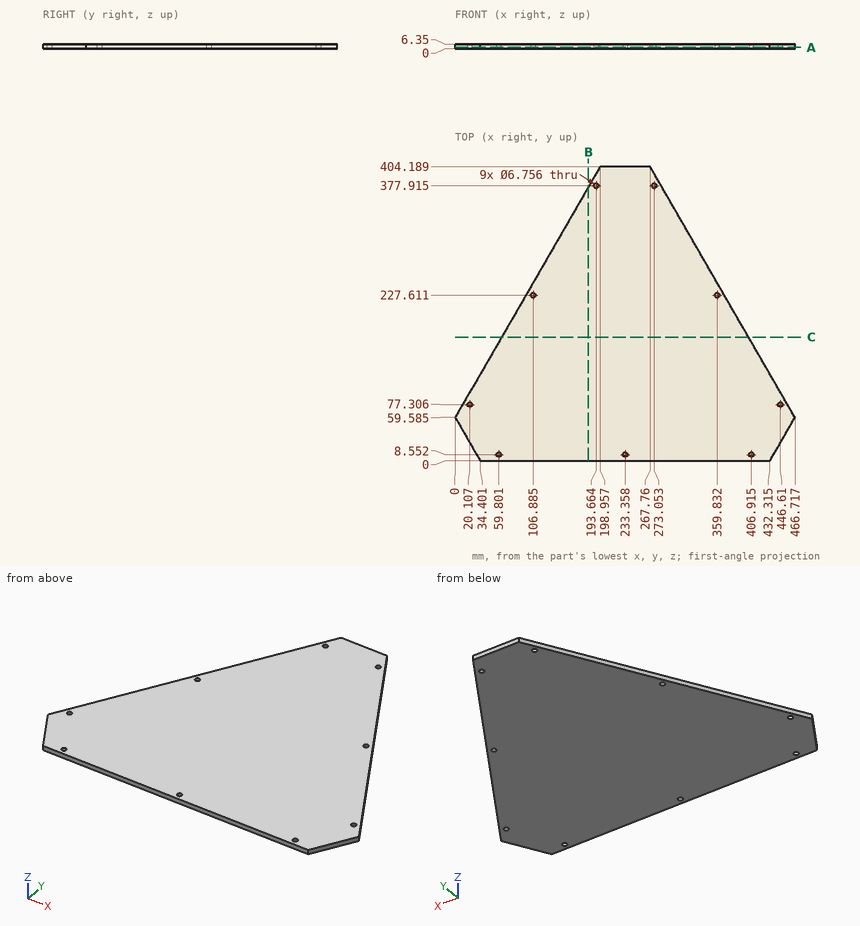
Drawing for the job (mm, zero at the part's lowest x, y, z). Give positions to 0.01 mm unless a question says otherwise; leave off trailing zeros. Loops run counter-clockwise (first coordinate to the right, second up) from the corner with the lowest first, then second, coordinate; pieces in that order, holes last. Notation, with made-up numbers: M 75.25,67 L 131.25,67 A26 cw 131.25,106 Z; hole C -34,67 d8. An arc over 180 degrees is marked long. Use one line per item in the form item = value.
Item 1: Slice it at B-B (x = 183). List the corners of the cut face in (y, z), plus the area to 3 significant figures.
Determined:
outline = M 0,0 L 376.55,0 L 376.55,6.35 L 0,6.35 Z
area = 2,390 mm2
Item 2: Drill centre lines: probe 1 along Y at (x, z) = (193, 5.75) (1 decimal); probe 2 along X at (y, z) = (142, 0.75) (1 decimal); probe 3 along X at (y, z) = (38, 1.25) (1 decimal). Where is each one in solid material? Low to high. Write a range as from..to.
Determined:
probe_1 = 0..374.6, 381.2..393.9
probe_2 = 47.6..419.1
probe_3 = 12.5..454.3
Item 3: Slice it at C-C (y = 170). List the corners of the cut face in (x, z), plus the area to 3 significant figures.
Determined:
outline = M 63.75,0 L 402.97,0 L 402.97,6.35 L 63.75,6.35 Z
area = 2,150 mm2
Item 4: Slice it at A-A (z = 1.75). Count the separate pieces of the cut face and the enclosed holes in it, plus the area to 3 significant figures.
Determined:
separate_pieces = 1
enclosed_holes = 9
area = 118,000 mm2
Item 5: Flat gauge pin, fed straight in: pin 1 (3 mm diameter, centred on x = 316, z = 1, fed in from +Y) (1 decimal). Where does the tip first touch, or does it go through?
Determined:
pin_1 = 323.2
